For this review, take the finished solid that the model builds, in its own axes (mm). A direction names the side the tool comes from. Coordinates: 2 decimals unless noted, no trailing zeros. Order: outer loops, then holes, each group sorted by start corner. A loop starts at its lowest first (then second) coordinate and runs counter-clockwise, first axis right, second up. Notation, with made-up numbers: (74.25, 57.5) -> (93.25, 57.5) arc R18 ccw to (93.25, 72.5) -> close; hole circle Ø1 at (58, -14). An arc over 180 degrees is marked (long way). Write item = value, one per line. Start each with the question number.
1) Consider section A-A on y = -13.5. Give the boundary of the cut face in (x, z).
2) Wall thickness on probe 1 along X at (y, z) = (-12.75, 9.75); probe 2 along Y at (x, z) = (1, -4) (3 decimals); probe 3 along Z at (x, y) = (-47.5, -9): over which ranges is each line inside the solid? List them lowest first. Write a range as [from, to].
3) Consider section C-C on z = 15. Give the boundary of the cut face in (x, y) (3 decimals).
4) Insertion check: pin 1 Ø12 at (x, z) = (-11.5, 15.5) entering from -Y (3 decimals); pin 2 Ø1.9 at (x, y) = (20, -5.5) entering from -Z; pin 3 Ø7 at (y, z) = (-10.5, 7) entering from +X. Each pin has a flat end and moves straight along its axis. Give the tip position at first contact, or say it passes through.
5) Consider section D-D on y = -7.5. Give the boundary of the cut face in (x, z), and give its area (3 significant figures).
6) Draft analysis for pull direction X (two halves, no side actions). For faces 4 (the face through (-16, -3.175, 5)), 5 (the face through (-51, -17.145, 11)), 6 (the face through (29.485, -2, 4)), state which applies: +X half, -X half, draft (parallel to the pull), parting line (faces both ways), or undercut.
7) Machinability: for faces 1 (the face through (-53.7, -12, 12)), 2 (the face through (16.15, -12, 12)), 3 (the face through (19, -7, 10.301)), which of the approach directions +Z, -Z, +X, -X, +Y, -Y give a long, thin tool a straight path to every point of the face, cutting with its end or side? Answer none if there is none.
8) Consider section B-B on z = 5.25. Give the boundary of the cut face in (x, y) (3 decimals).
from build123d import *

# Parameters (mm, degrees)
F0_W     = 90.17
F0_H     = 28.702
F1_DEPTH = 3.175
F2_W     = 6.35
F2_H     = 8.382
F3_DEPTH = 7.62
F4_W     = 6.35
F4_H     = 6.35
F5_DEPTH = 16.51


with BuildPart() as f1:
    # F0 (on Front) → F1 (new body)
    with BuildSketch(Plane.XZ):
        with Locations((-15.599873, 4.331834)):
            Rectangle(F0_W, F0_H)
    extrude(amount=F1_DEPTH)

    # F2 (on face) → F3 (join)
    with BuildSketch(Plane.XZ.offset(3.175)):
        with Locations((-50.524873, 14.491834)):
            Rectangle(F2_W, F2_H)
        with Locations((19.325127, 14.491834)):
            Rectangle(F2_W, F2_H)
    extrude(amount=F3_DEPTH)

    # F4 (on face) → F5 (join)
    with BuildSketch(Plane.XY.offset(18.682834)):
        with Locations((-50.524873, -13.97)):
            Rectangle(F4_W, F4_H)
        with Locations((19.325127, -13.97)):
            Rectangle(F4_W, F4_H)
    extrude(amount=-F5_DEPTH)


solid = f1.part
Answer sheet:
q1.outline = (-53.7, 2.17) -> (-47.35, 2.17) -> (-47.35, 18.68) -> (-53.7, 18.68) -> close; (16.15, 2.17) -> (22.5, 2.17) -> (22.5, 18.68) -> (16.15, 18.68) -> close
q2.probe_1 = [-53.7, -47.35], [16.15, 22.5]
q2.probe_2 = [-3.175, 0]
q2.probe_3 = [10.3, 18.68]
q3.outline = (-60.685, -3.175) -> (-53.7, -3.175) -> (-53.7, -17.145) -> (-47.35, -17.145) -> (-47.35, -3.175) -> (16.15, -3.175) -> (16.15, -17.145) -> (22.5, -17.145) -> (22.5, -3.175) -> (29.485, -3.175) -> (29.485, 0) -> (-60.685, 0) -> close
q4.pin_1 = -3.175
q4.pin_2 = 10.3
q4.pin_3 = 22.5
q5.outline = (-53.7, 10.3) -> (-47.35, 10.3) -> (-47.35, 18.68) -> (-53.7, 18.68) -> close; (16.15, 10.3) -> (22.5, 10.3) -> (22.5, 18.68) -> (16.15, 18.68) -> close
q5.area = 106 mm2
q6.face_4 = undercut
q6.face_5 = draft
q6.face_6 = +X half
q7.face_1 = +Z, -Z, -X, -Y
q7.face_2 = +Z, -Z, -Y
q7.face_3 = -Z, +X, -X
q8.outline = (-60.685, -3.175) -> (29.485, -3.175) -> (29.485, 0) -> (-60.685, 0) -> close; (-53.7, -17.145) -> (-47.35, -17.145) -> (-47.35, -10.795) -> (-53.7, -10.795) -> close; (16.15, -17.145) -> (22.5, -17.145) -> (22.5, -10.795) -> (16.15, -10.795) -> close
